Geometry: final body of the model. Coordinates: model frame, mm. Face numbers are marked on the shaded views. Round coordinates to 2 decimals unless told otherwise and drop trailing zeros. Write each loop counter-clockwise with the first axis right and the second up, starting at its lowest first coordinate (ties: lowest second). Pieces come first, ordered by that corner, then holes. Notation, with made-up numbers: (28, 13) -> (40, 13) arc R27 ccw to (40, 36) -> close; hole circle Ø2 at (58.5, 11). An arc over 180 degrees is marked (long way). One line per item, written item: value. Start each with the question number.
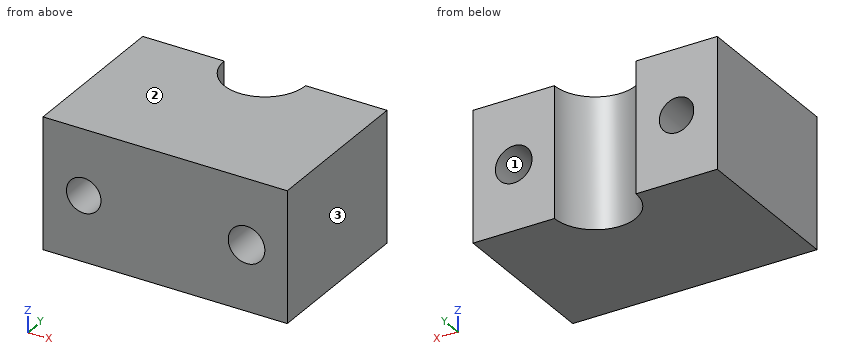
from build123d import *

# Parameters (mm, degrees)
SKETCH_W        = 30
SKETCH_H        = 16
PAD_DEPTH       = 20
SKETCH001_R     = 5
POCKET_DEPTH    = 16.001
SKETCH002_R     = 2.117093
SKETCH002_R_2   = 2.25
POCKET001_DEPTH = 20.001


with BuildPart() as part:
    # Sketch → Pad (new body)
    with BuildSketch(Plane.XZ):
        Rectangle(SKETCH_W, SKETCH_H)
    extrude(amount=PAD_DEPTH)

    # Sketch001 → Pocket (cut, through all)
    with BuildSketch(Plane(origin=(0, 0, 8), x_dir=(-1, 0, 0), z_dir=(0, 0, 1))):
        Circle(SKETCH001_R)
    extrude(amount=-POCKET_DEPTH, mode=Mode.SUBTRACT)

    # Sketch002 → Pocket001 (cut, through all)
    with BuildSketch(Plane(origin=(0, 0, 0), x_dir=(1, 0, 0), z_dir=(0, 1, 0))):
        with Locations((-10, 0)):
            Circle(SKETCH002_R)
        with Locations((10, 0)):
            Circle(SKETCH002_R_2)
    extrude(amount=-POCKET001_DEPTH, mode=Mode.SUBTRACT)


solid = part.part
(1) Section query B-B (y = -2.25). Output: boundary loops of the cut face in (x, z).
(2) Pull-direction query (Z, two-part tool) for the marked faces 1, 2 and 3; classes: pulls with the +Z half, pulls with the -Z half, needs draft (parallel to the pull), parting line crosses it, or undercut.
(3) Section query D-D (y = -9.5). Output: boundary loops of the cut face in (x, z).
(4) Section query A-A (x = -10). Output: boundary loops of the cut face in (y, z).
(5) Line query: probe 1 along X at (y, z) = (-5.5, 0); probe 2 along Z at (x, y) = (-10, -9); probe 3 along X at (y, z) = (-16.25, -1.5). Output: solid intervals per line, ascending.
(6) Section query C-C (z = 0). Output: boundary loops of the cut face in (x, y), and give its area (3 significant figures).
Results list:
1. outline: (-15, -8) -> (-4.47, -8) -> (-4.47, 8) -> (-15, 8) -> close; (4.47, -8) -> (15, -8) -> (15, 8) -> (4.47, 8) -> close; hole circle Ø4.23 at (-10, 0); hole circle Ø4.5 at (10, 0)
2. face 1: undercut
2. face 2: pulls with the +Z half
2. face 3: needs draft
3. outline: (-15, -8) -> (15, -8) -> (15, 8) -> (-15, 8) -> close; hole circle Ø4.23 at (-10, 0); hole circle Ø4.5 at (10, 0)
4. outline: (-20, -8) -> (0, -8) -> (0, -2.12) -> (-20, -2.12) -> close; (-20, 2.12) -> (0, 2.12) -> (0, 8) -> (-20, 8) -> close
5. probe 1: x = -15 to -12.12, -7.88 to 7.75, 12.25 to 15
5. probe 2: z = -8 to -2.12, 2.12 to 8
5. probe 3: x = -15 to -11.49, -8.51 to 8.32, 11.68 to 15
6. outline: (-15, -20) -> (-12.12, -20) -> (-12.12, 0) -> (-15, 0) -> close; (-7.88, -20) -> (7.75, -20) -> (7.75, 0) -> (5, 0) arc R5 cw to (-5, 0) -> (-7.88, 0) -> close; (12.25, -20) -> (15, -20) -> (15, 0) -> (12.25, 0) -> close
6. area: 386 mm^2
